Build history of the part. All positions in model axes, mm. Round coordinates to 2 decimals unless told otherwise and drop trailing zeros. Loops run counter-clockwise (first coordinate to the right, second up) from the corner with the lowest first, then second, coordinate; pieces in that order, holes last. Notation, with made-up numbers: (69.5, 3.5) -> (107.5, 3.5) arc R20 ccw to (107.5, 18.5) -> close; hole circle Ø1 at (-13, 63). An arc over 180 degrees is marked (long way). Put each result on its own line as item: value. Start each with the question number.
```python
from build123d import *

# Parameters (mm, degrees)
SKETCH2_W                 = 57.15
SKETCH2_H                 = 152.4
BOSS_EXTRUDE1_DEPTH       = 6.35
F_8_CLEARANCE_HOLE1_D     = 4.9149
F_8_CLEARANCE_HOLE1_DEPTH = 9.191415072
F_8_CLEARANCE_HOLE1_TIP   = 1.476584928


with BuildPart() as part:
    # Sketch2 → Boss-Extrude1 (new body)
    with BuildSketch(Plane.XY):
        with Locations((28.575, 76.2)):
            Rectangle(SKETCH2_W, SKETCH2_H)
    extrude(amount=BOSS_EXTRUDE1_DEPTH)

    # #8 Clearance Hole1
    with Locations(Plane.XY.offset(6.35)):
        with Locations((19.05, 9.525), (38.1, 9.525), (19.05, 142.875), (38.1, 142.875), (13.843, 76.2), (43.307, 76.2)):
            Hole(F_8_CLEARANCE_HOLE1_D / 2, depth=F_8_CLEARANCE_HOLE1_DEPTH)
            with Locations((0, 0, -(F_8_CLEARANCE_HOLE1_DEPTH + F_8_CLEARANCE_HOLE1_TIP / 2))):  # 118° drill point
                Cone(0, F_8_CLEARANCE_HOLE1_D / 2, F_8_CLEARANCE_HOLE1_TIP, mode=Mode.SUBTRACT)


solid = part.part
```
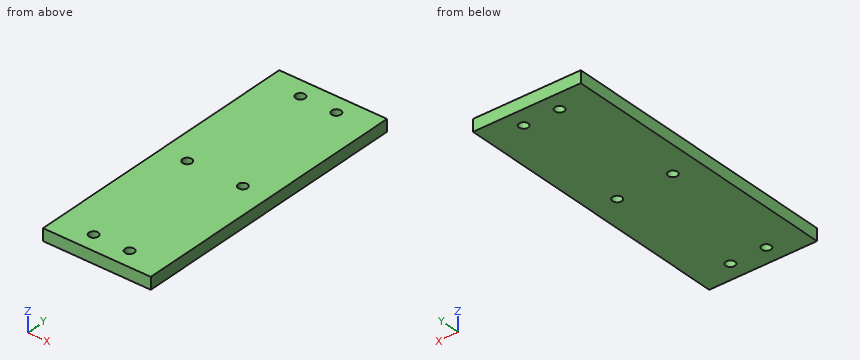
Item 1: Cut at A-A on y = 76.2. Write the cut outline in (x, z).
Item 2: Cut at B-B on x = 19.05. Write the cut outline in (y, z), then the cut area to 3 significant figures.
Item 3: Cut at C-C on x = 43. Write the cut outline in (y, z), then the cut area to 3 significant figures.
Item 4: Wall check: line 1 (Y direction, x = 19.05, z = 4); line 2 (X direction, y = 143, z = 2); line 3 (Y direction, x = 13.5, z = 2.5). Give the ranges that are in metal, low to high. Write a range as from..to.
Ans:
1. outline: (0, 0) -> (11.39, 0) -> (11.39, 6.35) -> (0, 6.35) -> close; (16.3, 0) -> (40.85, 0) -> (40.85, 6.35) -> (16.3, 6.35) -> close; (45.76, 0) -> (57.15, 0) -> (57.15, 6.35) -> (45.76, 6.35) -> close
2. outline: (0, 0) -> (7.07, 0) -> (7.07, 6.35) -> (0, 6.35) -> close; (11.98, 0) -> (140.42, 0) -> (140.42, 6.35) -> (11.98, 6.35) -> close; (145.33, 0) -> (152.4, 0) -> (152.4, 6.35) -> (145.33, 6.35) -> close
2. area: 905 mm2
3. outline: (0, 0) -> (73.76, 0) -> (73.76, 6.35) -> (0, 6.35) -> close; (78.64, 0) -> (152.4, 0) -> (152.4, 6.35) -> (78.64, 6.35) -> close
3. area: 937 mm2
4. line 1: y = 0..7.07, 11.98..140.42, 145.33..152.4
4. line 2: x = 0..16.6, 21.5..35.65, 40.55..57.15
4. line 3: y = 0..73.77, 78.63..152.4
